Source: three-view drawing plus pictorial views. Frame: mm from the lowest corner of the part. A direction names the side the tool comes from. Give positions to 0.01 mm unless a question says otherwise; leave off trailing zeros. Loops run counter-clockwise (first coordinate to the right, second up) from the corner with the lowest first, then second, coordinate; pieces in that order, holes last. Notation, with made-up numbers: M -18,17 L 6,17 A29 ccw 6,40 Z; hole C -18,-29.5 d7. An arc over 180 degrees is marked long. Put each result on its own line as item: value. Start each with the question number.
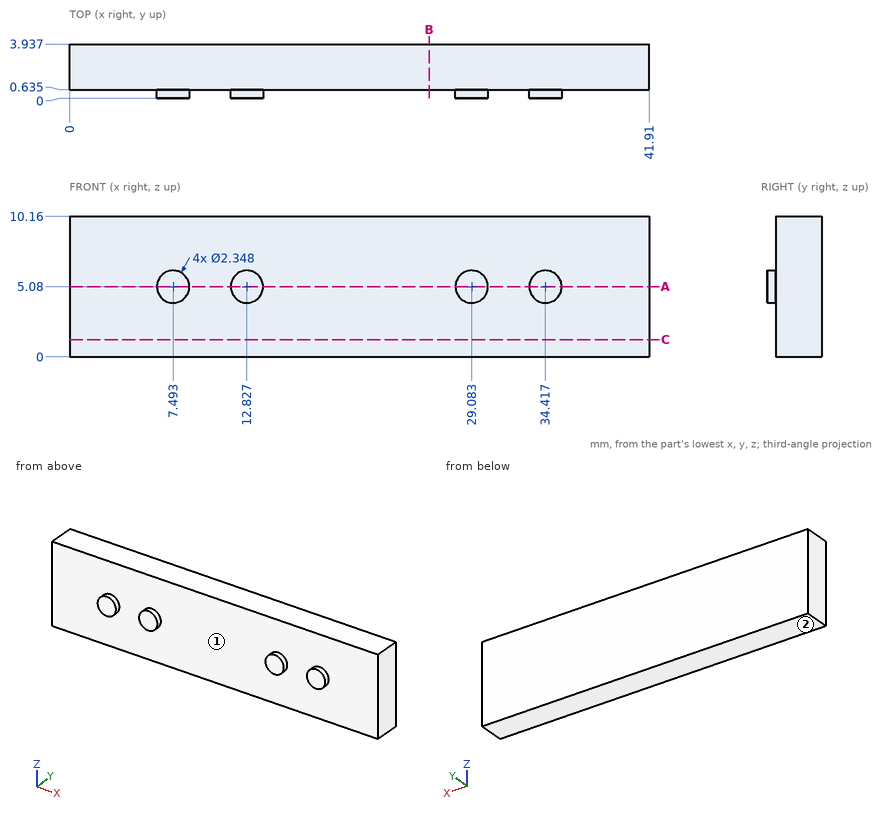
1. Set-up query: the marked faces 1 and 2. Return all of +Z, -Z, +X, -X, +Y, -Y with unobstructed straight access to the full face (end or side cutting, diameter ignored); none if empty.
2. Section C-C, the plane z = 1.25. Output: boundary loops of the cut face in (x, y) (3 decimals), plus the area to 3 significant figures.
3. Contact query for flat-ended pins moving along their axis: pin 1 (4 mm diameter, centred on x = 29, z = 5, fed in from -Y); pin 2 (1 mm diameter, centred on x = 12, z = 7.5, fed in from -Y) (3 decimals). Output: stop coordinate, or through.
4. Ray query, line 1 (Y direction, x = 24, z = 4.5) (3 decimals). Return the intervals inside material, ascending.
5. Section A-A, the plane z = 5.08. Output: boundary loops of the cut face in (x, y) (3 decimals), plus the area to 3 significant figures.
6. Section B-B, the plane x = 26. Output: boundary loops of the cut face in (y, z) (3 decimals).
Results found:
1. face 1: -Y
1. face 2: -Z, +X, -X, +Y, -Y
2. outline: M 0,0.635 L 41.91,0.635 L 41.91,3.937 L 0,3.937 Z
2. area: 138 mm²
3. pin 1: y = 0
3. pin 2: y = 0.635
4. line 1: 0.635 to 3.937
5. outline: M 0,0.635 L 6.319,0.635 L 6.319,0 L 8.667,0 L 8.667,0.635 L 11.653,0.635 L 11.653,0 L 14.001,0 L 14.001,0.635 L 27.909,0.635 L 27.909,0 L 30.257,0 L 30.257,0.635 L 33.243,0.635 L 33.243,0 L 35.591,0 L 35.591,0.635 L 41.91,0.635 L 41.91,3.937 L 0,3.937 Z
5. area: 144 mm²
6. outline: M 0.635,0 L 3.937,0 L 3.937,10.16 L 0.635,10.16 Z
